CAD build for the part. Positions are in the model's coordinates, mm. Face numbers are marked on the shaded views. A direction names the side the tool comes from. Round coordinates to 2 decimals unless told otherwise and drop trailing zeros. Write each loop counter-clockwise with the first axis right and the second up, starting at its lowest first coordinate (ties: lowest second). Pieces come first, ordered by that corner, then holes. Notation, with made-up numbers: (-22.75, -0.75) - (33.25, -0.75) arc R13 cw to (33.25, 5.25) - close; hole circle Ø10 at (-15.5, 83.25). An arc over 180 degrees is marked (long way). Answer in a Markdown table with one row per item.
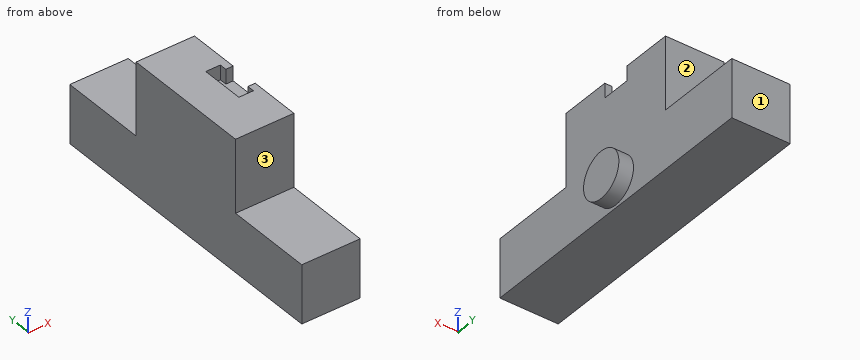
```python
from build123d import *

# Parameters (mm, degrees)
F0_W     = 20
F0_H     = 45
F1_DEPTH = 45
F3_DEPTH = 5
F4_R     = 8
F5_DEPTH = 5
F6_W     = 20
F6_H     = 20
F7_DEPTH = 30
F8_W     = 20
F8_H     = 20
F9_DEPTH = 30


with BuildPart() as f1:
    # F0 (on Top) → F1 (new body)
    with BuildSketch(Plane.XY):
        with Locations((-10, 22.5)):
            Rectangle(F0_W, F0_H)
    extrude(amount=F1_DEPTH)

    # F2 (on face) → F3 (cut)
    with BuildSketch(Plane.XY.offset(45)):
        Polygon((0, 17.5), (0, 27.5), (-2.5, 27.5), (-2.5, 30), (-7.5, 30), (-7.5, 15), (-2.5, 15), (-2.5, 17.5), align=None)
    extrude(amount=-F3_DEPTH, mode=Mode.SUBTRACT)

    # F4 (on face) → F5 (join)
    with BuildSketch(Plane.YZ):
        with Locations((22.5, 9)):
            Circle(F4_R)
    extrude(amount=F5_DEPTH)

    # F6 (on face) → F7 (join)
    with BuildSketch(Plane.XZ):
        with Locations((-10, 10)):
            Rectangle(F6_W, F6_H)
    extrude(amount=F7_DEPTH)

    # F8 (on face) → F9 (join)
    with BuildSketch(Plane(origin=(0, 45, 0), x_dir=(-1, 0, 0), z_dir=(0, 1, 0))):
        with Locations((10, 10)):
            Rectangle(F8_W, F8_H)
    extrude(amount=F9_DEPTH)


solid = f1.part
```
Q1. Saw through at A-A on y = 22.5. List the corners of the cut face in (x, z).
Computed:
| item | result |
|---|---|
| outline | (-20, 0) - (0, 0) - (0, 1) - (5, 1) - (5, 17) - (0, 17) - (0, 40) - (-7.5, 40) - (-7.5, 45) - (-20, 45) - close |
Q2. Saw through at C-C on x = -8.75. List the corners of the cut face in (y, z), then the cut area to 4 significant figures.
Computed:
| item | result |
|---|---|
| outline | (-30, 0) - (75, 0) - (75, 20) - (45, 20) - (45, 45) - (0, 45) - (0, 20) - (-30, 20) - close |
| area | 3,225 mm2 |
Q3. Drill centre lines: line 1 (X direction, y = 58, z = 19); line 2 (Y direction, x = -9.25, z = 38); line 3 (Z direction, x = -7, y = -6.5). Where is each one in solid material? Low to high.
Computed:
| item | result |
|---|---|
| line 1 | x = -20 to 0 |
| line 2 | y = 0 to 45 |
| line 3 | z = 0 to 20 |
Q4. Flat gauge pins, fed straight in: pin 1 (4 mm diameter, centred on x = -4.5, z = 41.5, fed in from +Y); pin 2 (6 mm diameter, centred on x = -2, y = 22, fed in from +Z); pin 3 (3 mm diameter, centred on y = -9.5, z = 21, fed in from +X). Where does each tip first touch, or does it go through?
Computed:
| item | result |
|---|---|
| pin 1 | stops at y = 45 |
| pin 2 | stops at z = 40 |
| pin 3 | stops at x = 0 |
Q5. Saw through at D-D on y = 65.5. List the corners of the cut face in (x, z).
Computed:
| item | result |
|---|---|
| outline | (-20, 0) - (0, 0) - (0, 20) - (-20, 20) - close |
Q6. Saw through at B-B on z = 9. List the corners of the cut face in (x, y), then the cut area to 3 significant figures.
Computed:
| item | result |
|---|---|
| outline | (-20, -30) - (0, -30) - (0, 14.5) - (5, 14.5) - (5, 30.5) - (0, 30.5) - (0, 75) - (-20, 75) - close |
| area | 2,180 mm2 |
Q7. 3-axis set-ups, long thin cutter, end or side, ignore diameter. For the marked faces 1, 2 and 3: which of +Z, -Z, +X, -X, +Y, -Y reach the whole face in a straight line?
Computed:
| item | result |
|---|---|
| face 1 | +Z, -Z, +X, -X, +Y |
| face 2 | +Z, +X, -X, +Y |
| face 3 | +Z, +X, -X, -Y |
